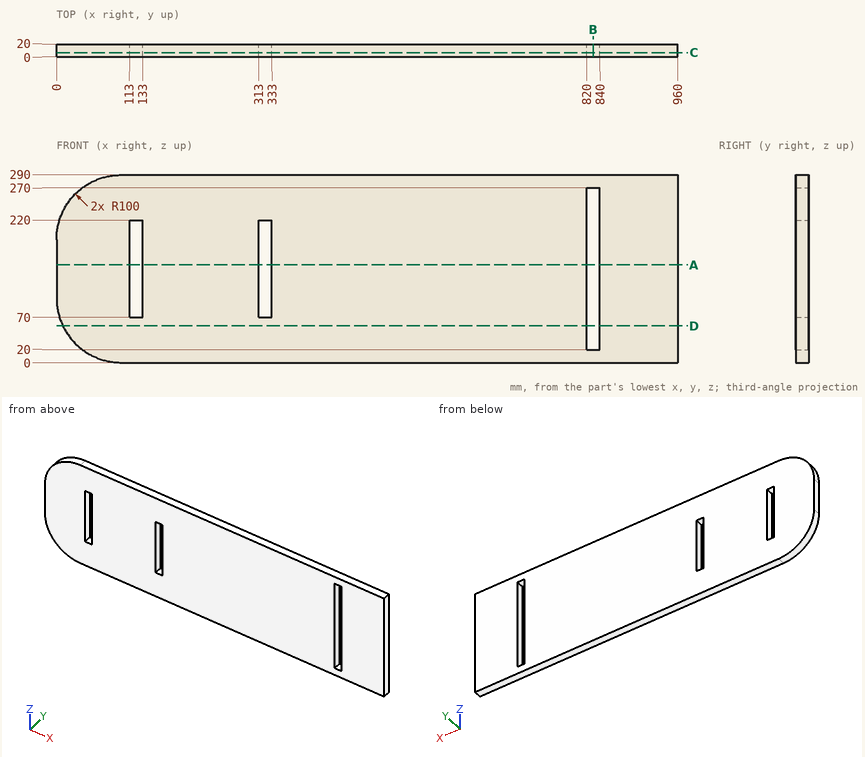
For this review, use the dimensioned drawing (mm, ordinates from the lowest corner) and the shaded views. Round coordinates to 2 decimals unless told otherwise and drop trailing zeros. Order: outer loops, then holes, each group sorted by start corner. A loop starts at its lowest first (then second) coordinate and runs counter-clockwise, first axis right, second up. Notation, with made-up numbers: (77.25, 42) -> (91.25, 42) arc R22 cw to (91.25, 75) -> close; hole circle Ø6 at (-5.5, -0.75). An arc over 180 degrees is marked (long way). Write item = value, one per line. Start each with the question number.
Item 1: Consider section B-B on x = 829.5. Write out the cut boundary in (y, z).
Item 2: For line 1 along X through (y, z) = (12.25, 194.5); line 2 along X through (y, z) = (17.75, 186); line 3 along Z through (x, y) = (116, 5), list the stretches that pass through material, from the lowest coordinate up.
Item 3: Consider section A-A on z = 151. Write out the cut boundary in (x, y), plus the area to 3 significant figures.
Item 4: Consider section C-C on y = 6.5. Write out the cut boundary in (x, z).
Item 5: Consider section D-D on z = 56.5. Write out the cut boundary in (x, y).
Conclusion:
q1.outline = (0, 0) -> (20, 0) -> (20, 20) -> (0, 20) -> close; (0, 270) -> (20, 270) -> (20, 290) -> (0, 290) -> close
q2.line_1 = 0.1 to 113, 133 to 313, 333 to 820, 840 to 960
q2.line_2 = 0 to 113, 133 to 313, 333 to 820, 840 to 960
q2.line_3 = 0 to 70, 220 to 290
q3.outline = (0, 0) -> (113, 0) -> (113, 20) -> (0, 20) -> close; (133, 0) -> (313, 0) -> (313, 20) -> (133, 20) -> close; (333, 0) -> (820, 0) -> (820, 20) -> (333, 20) -> close; (840, 0) -> (960, 0) -> (960, 20) -> (840, 20) -> close
q3.area = 18,000 mm2
q4.outline = (0, 100) arc R100 ccw to (100, 0) -> (960, 0) -> (960, 290) -> (100, 290) arc R100 ccw to (0, 190) -> close; hole (113, 70) -> (133, 70) -> (133, 220) -> (113, 220) -> close; hole (313, 70) -> (333, 70) -> (333, 220) -> (313, 220) -> close; hole (820, 20) -> (840, 20) -> (840, 270) -> (820, 270) -> close
q5.outline = (9.96, 0) -> (820, 0) -> (820, 20) -> (9.96, 20) -> close; (840, 0) -> (960, 0) -> (960, 20) -> (840, 20) -> close
